Here's how the part is built. I have some questions about the finished solid (model axes, mm). A direction names the side the tool comes from. Give positions to 0.01 mm unless a question says otherwise; leave off trailing zeros. Write each loop counter-clockwise with the first axis right and the second up, starting at its lowest first coordinate (ties: lowest second). Pieces come first, ordered by that corner, then holes. Notation, with made-up numbers: (77, 7) - (122, 7) arc R14 cw to (122, 17) - close; hole circle Ø6 at (35.5, 37). An arc over 180 degrees is marked (long way). One line per item, written item: value. Start each with the question number.
1) I'm going to push flat-ended pins straight in: P1, Ø1.5, axis at y = -1, z = 0, coming from the +X side; P2, Ø1, axis at x = -1, z = 0.5, coming from the -Y side. Where does each tip first touch, or does it pass through?
2) Imagine slicing it at A-A on y = 0. Write out the boundary of the cut face in (x, z) (3 decimals), plus the area to 4 significant figures.
3) Imagine slicing it at D-D on y = 18. Write out the boundary of the cut face in (x, z).
4) We'd pull the mould along X, two halves only. Please class faces 4 (the flat face through (4, 35, 0)), 5 (the cylindrical face through (0, 2.6, 0)), 6 (the cylindrical face through (-0.014, 46.556, -0.021)): +X half, -X half, draft (parallel to the pull), parting line (faces both ways), or undercut.
5) Imagine slicing it at C-C on z = -0.45. Write out the boundary of the cut face in (x, y) (1 decimal).
6) Imagine slicing it at B-B on x = 0. Write out the boundary of the cut face in (y, z), plus the area to 3 significant figures.
7) Please list where these lines run through material, in increasing order: L1, parallel to X at y = 0, z = -1.3 (3 decimals); L2, parallel to Y at x = 4.5, z = 1.05; L3, parallel to X at y = 44, z = 0.2. Write a range as [from, to].
8) On a 3-axis mill with a long thin cutter (end or side, diameter ignored), from which of +Z, -Z, +X, -X, +Y, -Y can I reach the whole of each face in a straight line? I mean faces 1 (the flat face through (-4, 35, 0)), 2 (the flat face through (-1.525, 0, 0)), 3 (the flat face through (3.76, 41.23, 0.02)). Say none if no direction works.
from build123d import *

# Parameters (mm, degrees)
F0_R     = 5.4
F1_DEPTH = 1.5
F3_DEPTH = 1.5
F5_DEPTH = 3
F6_R     = 1


with BuildPart() as f1:
    # F0 (on Top) → F1 (new body, symmetric)
    with BuildSketch(Plane.XY):
        Circle(F0_R)
        with BuildLine():
            ThreePointArc((1.525, 2.1057955741), (2.3157072354, 1.1821590418), (2.6, 0))
            ThreePointArc((2.6, 0), (2.3157072354, -1.1821590418), (1.525, -2.1057955741))
            ThreePointArc((1.525, -2.1057955741), (0, -2.6), (-1.525, -2.1057955741))
            ThreePointArc((-1.525, -2.1057955741), (-2.6, 0), (-1.525, 2.1057955741))
            ThreePointArc((-1.525, 2.1057955741), (0, 2.6), (1.525, 2.1057955741))
        make_face(mode=Mode.SUBTRACT)
        with BuildLine():
            Line((-1.525, -2.1057955741), (-1.525, 2.1057955741))
            ThreePointArc((-1.525, 2.1057955741), (-2.6, 0), (-1.525, -2.1057955741))
        make_face()
        with BuildLine():
            ThreePointArc((1.525, -2.1057955741), (2.3157072354, -1.1821590418), (2.6, 0))
            ThreePointArc((2.6, 0), (2.3157072354, 1.1821590418), (1.525, 2.1057955741))
            Line((1.525, 2.1057955741), (1.525, -2.1057955741))
        make_face()
    extrude(amount=F1_DEPTH, both=True)

    # F2 (on Top) → F3 (join, symmetric)
    with BuildSketch(Plane.XY):
        Polygon((3.0802667684, 35), (0, 35), (-3.0802667684, 35), (-2, 4.0652072057), (0, 4.0652072057), (2, 4.0652072057), align=None)
    extrude(amount=F3_DEPTH, both=True)

    # F4 (on face) → F5 (join, through all)
    with BuildSketch(Plane.XY.offset(1.5)):
        Polygon((0, 47.5), (-7.5, 35), (-3.0802667684, 35), (3.0802667684, 35), (7.5, 35), align=None)
    extrude(amount=-F5_DEPTH)

    # F6
    f6_edges = [f1.edges().sort_by_distance(p)[0] for p in [
        (-7.5, 35, 0),
        (0, 47.5, 0),
        (7.5, 35, 0),
    ]]
    fillet(f6_edges, radius=F6_R)


solid = f1.part
Numbers:
1. P1: x = 5.39
1. P2: y = -5.38
2. outline: (-5.4, -1.5) - (-1.525, -1.5) - (-1.525, 1.5) - (-5.4, 1.5) - close; (1.525, -1.5) - (5.4, -1.5) - (5.4, 1.5) - (1.525, 1.5) - close
2. area: 23.25 mm^2
3. outline: (-2.49, -1.5) - (2.49, -1.5) - (2.49, 1.5) - (-2.49, 1.5) - close
4. face 4: draft
4. face 5: undercut
4. face 6: parting line
5. outline: (-6.6, 36.5) arc R1 ccw to (-5.7, 35) - (-3.1, 35) - (-2, 5) arc R5.4 ccw (long way) to (2, 5) - (3.1, 35) - (5.7, 35) arc R1 ccw to (6.6, 36.5) - (0.9, 46.1) arc R1 ccw to (-0.9, 46.1) - close; hole (-1.5, -2.1) arc R2.6 ccw to (1.5, -2.1) - (1.5, 2.1) arc R2.6 ccw to (-1.5, 2.1) - close
6. outline: (-5.4, -1.5) - (-2.6, -1.5) - (-2.6, 1.5) - (-5.4, 1.5) - close; (2.6, -1.5) - (46.56, -1.5) - (46.56, 1.5) - (2.6, 1.5) - close
6. area: 140 mm^2
7. L1: [-5.4, -1.525], [1.525, 5.4]
7. L2: [-2.98, 2.98], [35, 40]
7. L3: [-2.1, 2.1]
8. face 1: +Z, -Z, -X
8. face 2: +Z, -Z
8. face 3: +Z, -Z, +X, +Y
